Part model, mm, in its own coordinate system. A direction names the side the tool comes from. Round coordinates to 2 decimals unless told otherwise and drop trailing zeros. Order: outer loops, then holes, each group sorted by start corner. A loop starts at its lowest first (then second) coordinate and runs counter-clockwise, first axis right, second up. Notation, with made-up numbers: (-33, -6) - (-26, -6) arc R22 cw to (-26, 20) - close; hole circle Ø4 at (66.25, 43). An arc over 180 degrees is marked (long way). Answer as a JSON object with one key per item and string values.
```python
from build123d import *

# Parameters (mm, degrees)
ESQUISSE1_W             = 159
ESQUISSE1_H             = 106
BOSS_EXTRU_1_DEPTH      = 5
ENL_V_START             = -3
ESQUISSE3_R             = 5.5
ENL_V_MAT_EXTRU_2_DEPTH = 2.2
ESQUISSE4_W             = 109
ESQUISSE4_H             = 86
ENL_V_MAT_EXTRU_3_DEPTH = 6
ESQUISSE5_R             = 2
ENL_V_MAT_EXTRU_4_DEPTH = 6
CHANFREIN1_SIZE         = 2
CHANFREIN1_SIZE2        = 1.5071081
BOSS_EXTRU_2_START      = -5
BOSS_EXTRU_2_DEPTH      = 1
CONG_2_R                = 1


with BuildPart() as part:
    # Esquisse1 → Boss.-Extru.1 (new body)
    with BuildSketch(Plane.XY):
        with Locations((79.5, 53)):
            Rectangle(ESQUISSE1_W, ESQUISSE1_H)
    extrude(amount=BOSS_EXTRU_1_DEPTH)

    # Esquisse3 → Enlèv. mat.-Extru.2 (cut)
    with BuildSketch(Plane(origin=(0, 0, 0), x_dir=(-1, 0, 0), z_dir=(0, 0, -1)).offset(ENL_V_START)):
        with Locations((-13.75, 36)):
            Circle(ESQUISSE3_R)
        with Locations((-13.75, 96)):
            Circle(ESQUISSE3_R)
        with Locations((-145.25, 36)):
            Circle(ESQUISSE3_R)
        with Locations((-145.25, 96)):
            Circle(ESQUISSE3_R)
    extrude(amount=-ENL_V_MAT_EXTRU_2_DEPTH, mode=Mode.SUBTRACT)

    # Esquisse4 → Enlèv. mat.-Extru.3 (cut)
    with BuildSketch(Plane.XY.offset(5)):
        with Locations((79.5, 63)):
            Rectangle(ESQUISSE4_W, ESQUISSE4_H)
    extrude(amount=-ENL_V_MAT_EXTRU_3_DEPTH, mode=Mode.SUBTRACT)

    # Esquisse5 → Enlèv. mat.-Extru.4 (cut)
    with BuildSketch(Plane.XY.offset(5)):
        with Locations((15, 10)):
            Circle(ESQUISSE5_R)
        with Locations((144, 10)):
            Circle(ESQUISSE5_R)
        with Locations((12.5, 81)):
            Circle(ESQUISSE5_R)
        with Locations((146.5, 81)):
            Circle(ESQUISSE5_R)
        with Locations((79.5, 10)):
            Circle(ESQUISSE5_R)
    extrude(amount=-ENL_V_MAT_EXTRU_4_DEPTH, mode=Mode.SUBTRACT)

    # Chanfrein1
    chanfrein1_edges = [part.edges().sort_by_distance(p)[0] for p in [
        (13, 10, 5),
        (142, 10, 5),
        (10.5, 81, 5),
        (144.5, 81, 5),
        (77.5, 10, 5),
    ]]
    chanfrein1_side = [part.faces().sort_by_distance(p)[0] for p in [
        (1.910942176, 53, 5),
    ]]
    chamfer(chanfrein1_edges, length=CHANFREIN1_SIZE, length2=CHANFREIN1_SIZE2, reference=chanfrein1_side[0])

    # Esquisse2 → Boss.-Extru.2 (add)
    with BuildSketch(Plane(origin=(0, 0, 0), x_dir=(-1, 0, 0), z_dir=(0, 0, -1)).offset(BOSS_EXTRU_2_START)):
        Polygon((-11.75, 64), (-7.75, 64), (-7.75, 68), (-11.75, 68), (-11.75, 72), (-15.75, 72), (-15.75, 68), (-19.75, 68), (-19.75, 64), (-15.75, 64), (-15.75, 60), (-11.75, 60), align=None)
        Polygon((-143.25, 64), (-139.25, 64), (-139.25, 68), (-143.25, 68), (-143.25, 72), (-147.25, 72), (-147.25, 68), (-151.25, 68), (-151.25, 64), (-147.25, 64), (-147.25, 60), (-143.25, 60), align=None)
    extrude(amount=-BOSS_EXTRU_2_DEPTH)

    # Congé2
    cong_2_edges = [part.edges().sort_by_distance(p)[0] for p in [
        (11.75, 62, 6),
        (13.75, 60, 6),
        (15.75, 62, 6),
        (19.75, 66, 6),
        (17.75, 64, 6),
        (17.75, 68, 6),
        (15.75, 70, 6),
        (13.75, 72, 6),
        (11.75, 70, 6),
        (143.25, 70, 6),
        (145.25, 72, 6),
        (147.25, 70, 6),
        (149.25, 68, 6),
        (151.25, 66, 6),
        (149.25, 64, 6),
        (147.25, 62, 6),
        (145.25, 60, 6),
        (143.25, 62, 6),
        (141.25, 64, 6),
        (141.25, 68, 6),
        (139.25, 66, 6),
        (9.75, 68, 6),
        (7.75, 66, 6),
        (9.75, 64, 6),
    ]]
    fillet(cong_2_edges, radius=CONG_2_R - 0.0001)  # a hair under: the kernel refuses the full size


solid = part.part
```
Item 1: Cut at D-D (x = 79.5). Write the cut outline in (y, z).
Taken from the geometry:
{"outline": "(0, 0) - (8, 0) - (8, 3.49) - (6, 5) - (0, 5) - close; (12, 0) - (20, 0) - (20, 5) - (14, 5) - (12, 3.49) - close"}
Item 2: Two-plate mould, pull along Y, no slides. Class faces 1 (the flat face through (159, 52, 2)), 2 (the flat face through (14, 96, 3)), 3 (the conical face through (13.3, 8.7, 3.6)), 4 (the flat face through (79, 20, 3)): pulls with the +Y half, pulls with the -Y half, needs draft (parallel to the pull), parting line crosses it, or undercut.
Taken from the geometry:
{"face 1": "needs draft", "face 2": "undercut", "face 3": "undercut", "face 4": "pulls with the +Y half"}
Item 3: Cut at B-B (y = 96). Write the cut outline in (x, z), plus the area to 3 significant figures.
Taken from the geometry:
{"outline": "(0, 0) - (25, 0) - (25, 5) - (19.25, 5) - (19.25, 3) - (8.25, 3) - (8.25, 5) - (0, 5) - close; (134, 0) - (159, 0) - (159, 5) - (150.75, 5) - (150.75, 3) - (139.75, 3) - (139.75, 5) - (134, 5) - close", "area": "206 mm2"}
Item 4: Cut at C-C (z = 1.7). Write the cut outline in (x, y).
Taken from the geometry:
{"outline": "(0, 0) - (159, 0) - (159, 106) - (134, 106) - (134, 20) - (25, 20) - (25, 106) - (0, 106) - close; hole circle Ø4 at (12.5, 81); hole circle Ø4 at (15, 10); hole circle Ø4 at (79.5, 10); hole circle Ø4 at (144, 10); hole circle Ø4 at (146.5, 81)"}
Item 5: Drop flat-ended pins along their axis: P1, Ø17.5, axis at x = 13.75, y = 96, coming from the +Z side; P2, Ø1, axis at x = 119, z = 1.5, coming from the -Y side; P3, Ø3.5, axis at x = 146.5, y = 81, coming from the +Z side. Give the stop position or say it passes through.
Taken from the geometry:
{"P1": "z = 5", "P2": "y = 0", "P3": "through"}
Item 6: Probe L1, parallel to X at y = 96.5, z = 4.65; L2, parallel to X at y = 68.5, z = 1.05; L3, parallel to Z at x = 82, y = 16. List the from-to ranges inside material, lowest first. Write a range as from..to.
Taken from the geometry:
{"L1": "0..8.27, 19.23..25, 134..139.77, 150.73..159", "L2": "0..25, 134..159", "L3": "0..5"}
Item 7: Tool access for faces 5 (the cylindrical face through (150.745, 36.242, 3.986)), 6 (the flat face through (78, 0, 2)), 7 (the flat face through (134, 62, 3)): list every direction of +Z, -Z, +X, -X, +Y, -Y with a clear straight run to the whole face (end or side of a thin tool).
Taken from the geometry:
{"face 5": "+Z", "face 6": "+Z, -Z, +X, -X, -Y", "face 7": "+Z, -Z, +Y"}
Item 8: Cut at A-A (y = 81). Write the cut outline in (x, z), plus the area to 3 significant figures.
Taken from the geometry:
{"outline": "(0, 0) - (10.5, 0) - (10.5, 3.49) - (8.5, 5) - (0, 5) - close; (14.5, 0) - (25, 0) - (25, 5) - (16.5, 5) - (14.5, 3.49) - close; (134, 0) - (144.5, 0) - (144.5, 3.49) - (142.5, 5) - (134, 5) - close; (148.5, 0) - (159, 0) - (159, 5) - (150.5, 5) - (148.5, 3.49) - close", "area": "204 mm2"}
